```python
from build123d import *

# Parameters (mm, degrees)
F1_DEPTH = 15.3468120843
F2_R     = 0.540493976


with BuildPart() as f1:
    # F0 (on Top) → F1 (new body)
    with BuildSketch(Plane.XY):
        Polygon((-46.3772900403, 15.7230943441), (-46.3772900403, -33.35686028), (0, -33.35686028), (0, -9.8423212767), (-12.8479711711, -9.8423212767), (-12.8479711711, 0), (0, 0), (0, 15.7230943441), align=None)
    extrude(amount=F1_DEPTH)

    # F2
    f2_edges = [f1.edges().sort_by_distance(p)[0] for p in [
        (0, -21.599591, 15.346812),
        (0, 7.861547, 15.346812),
        (-12.847971, -4.921161, 15.346812),
        (-6.423986, -9.842321, 15.346812),
        (-12.847971, 0, 7.673406),
        (0, 0, 7.673406),
        (-6.423986, 0, 0),
        (-6.423986, 0, 15.346812),
        (-12.847971, -4.921161, 0),
    ]]
    fillet(f2_edges, radius=F2_R)


solid = f1.part
```
Input: part model. Units: mm. Frame: model coordinates. A direction names the side the tool comes from. Coordinates: 2 decimals unless noted, no trailing zeros. Write each loop counter-clockwise with the first axis right and the second up, starting at its lowest first coordinate (ties: lowest second). Pieces come first, ordered by that corner, then holes. Notation, with made-up numbers: (-37.5, 80.25) - (19.5, 80.25) arc R16 ccw to (19.5, 86.25) - close; hole circle Ø9 at (76, 6). An arc over 180 degrees is marked (long way). Put each result on its own line as item: value. Start each with the question number.
1) Cut plane A-A (x = -5.5). Return the cut outline in (y, z).
2) Cut plane C-C (y = -2.5). Return the cut outline in (x, z), plus the area to 3 significant figures.
3) Cut plane B-B (z = 6). Return the cut outline in (x, y), plus the area to 3 significant figures.
4) Mould query, pull axis Y, two halves, no side actions, for faces 1 (the face through (-23, 15.723, 8)), 2 (the face through (0, -22, 7)), 3 (the face through (-7, 0, 8)). Classes: pulls with the +Y half, pulls with the -Y half, needs draft (parallel to the pull), parting line crosses it, or undercut.
5) Reachability of faces 4 (the face through (-24, -33.357, 8)), 5 (the face through (-12.848, -5, 8)) from +Z, -Z, +X, -X, +Y, -Y: full face, straight path, thin tool, end or side. Return the list, or none.
6) Ray query, L1, parallel to Y at x = -3, z = 9.25; L2, parallel to Z at x = -11.5, y = -10. Return the intervals inside material, ascending.
Resolved:
1. outline: (-33.36, 0) - (-9.84, 0) - (-9.84, 14.81) arc R0.54 ccw to (-10.38, 15.35) - (-33.36, 15.35) - close; (0, 0.54) arc R0.54 ccw to (0.54, 0) - (15.72, 0) - (15.72, 15.35) - (0.54, 15.35) arc R0.54 ccw to (0, 14.81) - close
2. outline: (-46.38, 0) - (-13.39, 0) arc R0.54 ccw to (-12.85, 0.54) - (-12.85, 14.81) arc R0.54 ccw to (-13.39, 15.35) - (-46.38, 15.35) - close
2. area: 514 mm2
3. outline: (-46.38, -33.36) - (0, -33.36) - (0, -9.84) - (-12.85, -9.84) - (-12.85, -0.54) arc R0.54 cw to (-12.31, 0) - (-0.54, 0) arc R0.54 ccw to (0, 0.54) - (0, 15.72) - (-46.38, 15.72) - close
3. area: 2,150 mm2
4. face 1: pulls with the +Y half
4. face 2: needs draft
4. face 3: undercut
5. face 4: +Z, -Z, +X, -X, -Y
5. face 5: +Z, -Z, +X
6. L1: y = -33.36 to -9.84, 0 to 15.72
6. L2: z = 0 to 15.19
